Check sheet for the drawn part. Datum: minimum x, y, z corner. Units: mm. Give positions to 0.01 mm unless a question says otherwise; leave off trailing zeros. Order: outer loops, then holes, each group sorted by start corner. A loop starts at its lowest first (then second) coordinate and runs counter-clockwise, first axis right, second up. Notation, with made-up numbers: M 13.5,-22.5 L 71.5,-22.5 A20 ccw 71.5,2.5 Z; hole C 56,-23 d10. An arc over 180 degrees is marked long. Put each result on its own line as item: value. Start each with the question number.
Q1. Section check A-A on x = 133. Record the cut outline in (y, z).
Q2. Go/stop test with flat-tipped pins: pin 1 (6.5 mm diameter, centred on x = 17, y = 8, fed in from +Z); pin 2 (3 mm diameter, centred on x = 17, y = 72, fed in from -Z). Record where each tip stops, or that it passes through.
Q3. Section check B-B on z = 2.7. Record the cut outline in (x, y), then the cut area to 3 significant figures.
Q4. Material ranges on L1, parallel to Y at x = 17, z = 2.2; L2, parallel to Y at x = 88, z = 2.35; L3, parallel to X at y = 7, z = 3.5, recorded low to high.
Q5. Section check D-D on y = 44. Record the cut outline in (x, z), then the cut area to 3 significant figures.
Q6. Section check C-C on y = 8. Record the cut outline in (x, z).
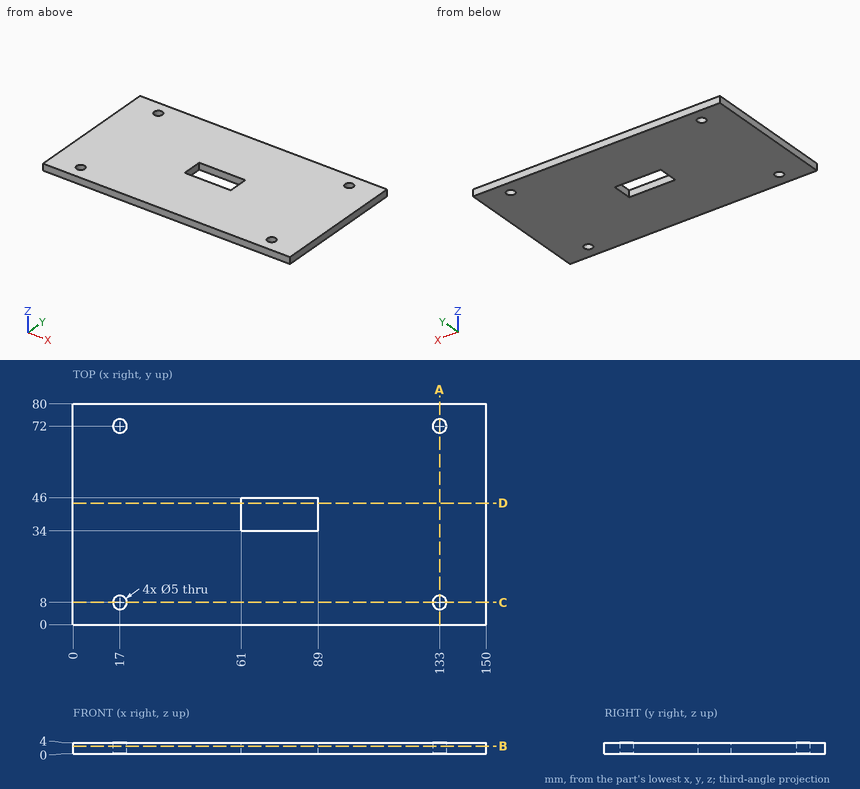
Results found:
1. outline: M 0,0 L 5.5,0 L 5.5,4 L 0,4 Z; M 10.5,0 L 69.5,0 L 69.5,4 L 10.5,4 Z; M 74.5,0 L 80,0 L 80,4 L 74.5,4 Z
2. pin 1: stops at z = 4
2. pin 2: passes through
3. outline: M 0,0 L 150,0 L 150,80 L 0,80 Z; hole C 17,8 d5; hole C 17,72 d5; hole M 61,34 L 89,34 L 89,46 L 61,46 Z; hole C 133,8 d5; hole C 133,72 d5
3. area: 11,600 mm^2
4. L1: y = 0 to 5.5, 10.5 to 69.5, 74.5 to 80
4. L2: y = 0 to 34, 46 to 80
4. L3: x = 0 to 14.71, 19.29 to 130.71, 135.29 to 150
5. outline: M 0,0 L 61,0 L 61,4 L 0,4 Z; M 89,0 L 150,0 L 150,4 L 89,4 Z
5. area: 488 mm^2
6. outline: M 0,0 L 14.5,0 L 14.5,4 L 0,4 Z; M 19.5,0 L 130.5,0 L 130.5,4 L 19.5,4 Z; M 135.5,0 L 150,0 L 150,4 L 135.5,4 Z
